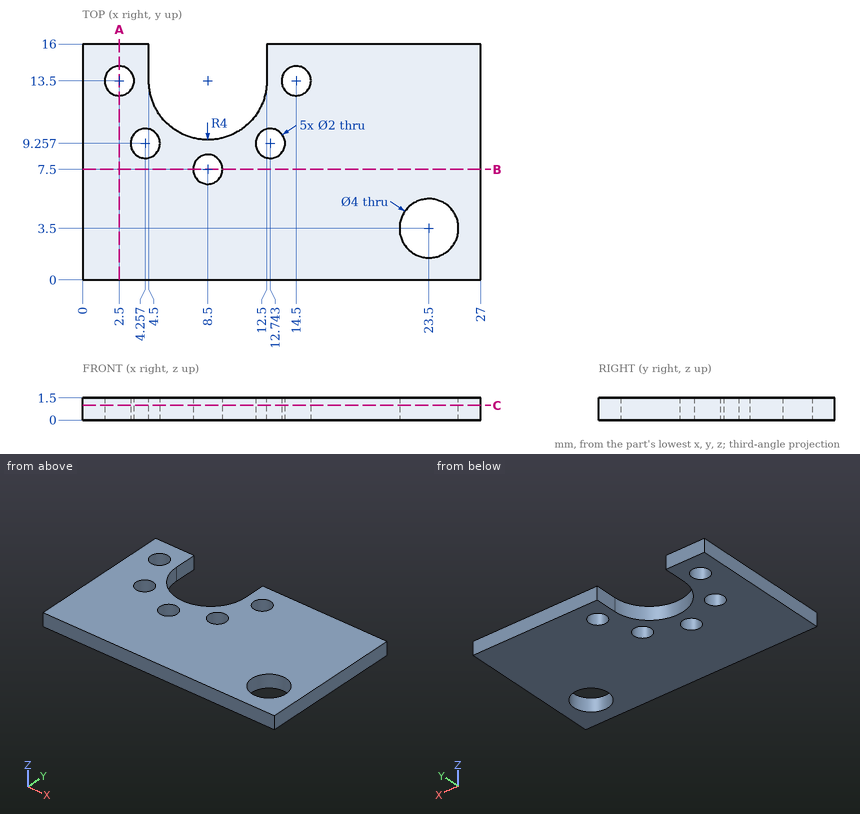
Input: dimensioned drawing with shaded views. Units: mm. Origin: part minimum x, y, z. Give positions to 0.01 mm unless a question says otherwise; leave off trailing zeros. Order: outer loops, then holes, each group sorted by start corner. A loop starts at its lowest first (then second) coordinate and runs counter-clockwise, first axis right, second up.
(1) Contact query for a flat-ended pin moving along its axis: P1, Ø5, axis at x = 6.5, y = 12.5, coming from the -Z side. Output: stop coordinate, or through.
(2) Section query C-C (z = 1). Return the cut outline in (x, y).
(3) Section query B-B (y = 7.5). Return the cut outline in (x, z), plus the area to 3 significant figures.
(4) Section query A-A (x = 2.5). Return the cut outline in (y, z), plus the area to 3 significant figures.
(5) Material intervals for line 1 along Y through (x, z) = (14.5, 1.25); line 2 along Y through (x, z) = (22, 0.1) (1 decimal); line 3 along X through (y, z) = (2, 0.65) (1 decimal), sorted ascending.
Outcome:
1. P1: stops at z = 0
2. outline: (0, 0) - (27, 0) - (27, 16) - (12.5, 16) - (12.5, 13.5) arc R4 cw to (4.5, 13.5) - (4.5, 16) - (0, 16) - close; hole circle Ø2 at (2.5, 13.5); hole circle Ø2 at (4.26, 9.26); hole circle Ø2 at (8.5, 7.5); hole circle Ø2 at (12.74, 9.26); hole circle Ø2 at (14.5, 13.5); hole circle Ø4 at (23.5, 3.5)
3. outline: (0, 0) - (7.5, 0) - (7.5, 1.5) - (0, 1.5) - close; (9.5, 0) - (27, 0) - (27, 1.5) - (9.5, 1.5) - close
3. area: 37.5 mm2
4. outline: (0, 0) - (12.5, 0) - (12.5, 1.5) - (0, 1.5) - close; (14.5, 0) - (16, 0) - (16, 1.5) - (14.5, 1.5) - close
4. area: 21.0 mm2
5. line 1: y = 0 to 12.5, 14.5 to 16
5. line 2: y = 0 to 2.2, 4.8 to 16
5. line 3: x = 0 to 22.2, 24.8 to 27
